from build123d import *

# Parameters (mm, degrees)
SKETCH_1_R          = 10
EXTRUDE_1_DEPTH     = 2
SKETCH_3_R          = 7.5
CUT_EXTRUDE_1_DEPTH = 12.5
SKETCH_5_R          = 1
SKETCH_5_W          = 2
SKETCH_5_H          = 2
EXTRUDE_5_DEPTH     = 1.5


with BuildPart() as part:
    # 草图1 → 凸台-拉伸1 (new body)
    with BuildSketch(Plane(origin=(0, 0, 0), x_dir=(0, 0, -1), z_dir=(1, 0, 0))):
        Circle(SKETCH_1_R)
    extrude(amount=EXTRUDE_1_DEPTH)

    # 草图3 → 切除-拉伸1 (cut)
    with BuildSketch(Plane(origin=(2, 0, 0), x_dir=(0, 0, -1), z_dir=(1, 0, 0))):
        Circle(SKETCH_3_R)
    extrude(amount=-CUT_EXTRUDE_1_DEPTH, mode=Mode.SUBTRACT)

    # 草图5 → 凸台-拉伸5 (add)
    with BuildSketch(Plane(origin=(2, 0, 0), x_dir=(0, 0, -1), z_dir=(1, 0, 0))):
        with Locations((0, 8.5)):
            Circle(SKETCH_5_R)
        with Locations((7.361215932, -4.25)):
            Circle(SKETCH_5_R)
        with Locations((-7.361215932, -4.25)):
            Circle(SKETCH_5_R)
        with Locations((-5.629165125, -3.25)):
            Circle(SKETCH_5_R)
        with Locations((0, 6.5)):
            Circle(SKETCH_5_R)
        with Locations((5.629165125, -3.25)):
            Circle(SKETCH_5_R)
        Polygon((-7.861215932, -3.383974596), (-6.129165125, -2.383974596), (-5.129165125, -4.116025404), (-6.861215932, -5.116025404), align=None)
        with Locations((0, 7.5)):
            Rectangle(SKETCH_5_W, SKETCH_5_H)
        Polygon((6.129165125, -2.383974596), (7.861215932, -3.383974596), (6.861215932, -5.116025404), (5.129165125, -4.116025404), align=None)
    extrude(amount=EXTRUDE_5_DEPTH)


solid = part.part
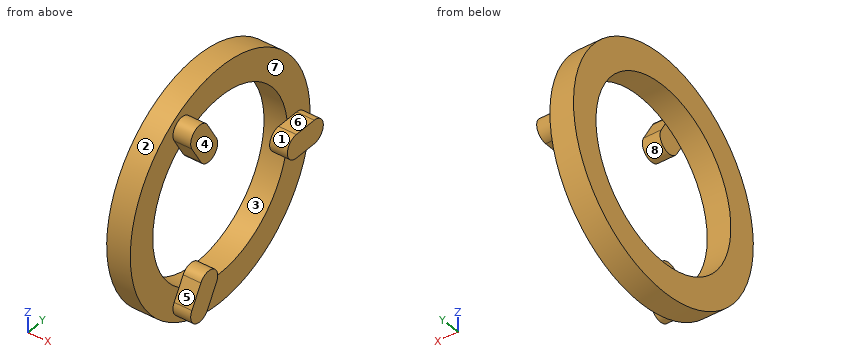
Part model, mm, in its own coordinate system. Face numbers are marked on the shaded views. A direction names the side the tool comes from. Coordinates: 2 decimals unless noted, no trailing zeros. Loops run counter-clockwise (first coordinate to the right, second up) from the corner with the lowest first, then second, coordinate; pieces in that order, holes last. Notation, with made-up numbers: (69.25, 55) -> (114.25, 55) arc R27 cw to (114.25, 76) -> close; hole circle Ø4 at (84.25, 61). An arc over 180 degrees is marked (long way). Use a Markdown table: item, result. Add a question column.
Item 1: Band-saw the part on D-D on x = 1.4. Write the cut outline in (y, z), plus the area to 3 significant figures.
Item 2: Band-saw the part on B-B on x = 3.1. Write the cut outline in (y, z), plus the area to 3 significant figures.
Item 3: Pull direction Y, two halves, no side cores. Call the marked faces 1, 2 and 3: +Y half, -Y half, draft (parallel to the pull), parting line (faces both ways), or undercut.
Item 4: Band-saw the part on C-C on z = 0. Write the cut outline in (x, y), plus the area to 3 significant figures.
Item 5: Probe probe 1 along Y at (x, z) = (1.05, 0); probe 2 along Z at (x, y) = (0.8, 2.5). List the from-to ranges inside material, lowest first.
Item 6: Which spindle directions (+Z, -Z, +X, -X, +Y, -Y) get a long thin tool onto all of the face, cutting with end or side? Do the marked faces 4, 5, 6, 7 and 8. Say none if no direction does.
Item 7: Band-saw the part on A-A on y = 0. Write the cut outline in (x, z), plus the area to 3 significant figures.
Item 8: Flat gauge pins, fed straight in: P1, Ø1.2, axis at x = 3, y = 7, coming from the +Z side; P2, Ø1.2, axis at y = -3, z = -6, coming from the -X side; P3, Ø1, axis at x = 1.5, z = 2.5, coming from the -Y side. Where does each tip first touch, or does it go through?
Geometry says:
| question | item | result |
|---|---|---|
| 1 | outline | circle Ø20 at (0, 0); hole circle Ø15 at (0, 0) |
| 1 | area | 137 mm² |
| 2 | outline | (-5.12, -6.86) arc R1 ccw to (-3.38, -7.86) -> (-2.38, -6.13) arc R1 ccw to (-4.12, -5.13) -> close; (-5.12, 6.86) -> (-4.12, 5.13) arc R1 ccw to (-2.38, 6.13) -> (-3.38, 7.86) arc R1 ccw to start; (6.5, -1) -> (8.5, -1) arc R1 ccw to (8.5, 1) -> (6.5, 1) arc R1 ccw to start |
| 2 | area | 21.4 mm² |
| 3 | face 1 | -Y half |
| 3 | face 2 | parting line |
| 3 | face 3 | undercut |
| 4 | outline | (0, -10) -> (2, -10) -> (2, -7.5) -> (0, -7.5) -> close; (0, 7.5) -> (2, 7.5) -> (2, 5.5) -> (3.5, 5.5) -> (3.5, 9.5) -> (2, 9.5) -> (2, 10) -> (0, 10) -> close |
| 4 | area | 16.0 mm² |
| 5 | probe 1 | -10 to -7.5, 7.5 to 10 |
| 5 | probe 2 | -9.68 to -7.07, 7.07 to 9.68 |
| 6 | face 4 | +Z, -Z, +X, +Y, -Y |
| 6 | face 5 | +X, -Y |
| 6 | face 6 | +Z, +X, +Y, -Y |
| 6 | face 7 | +X |
| 6 | face 8 | +X, -X |
| 7 | outline | (0, -10) -> (2, -10) -> (2, -7.5) -> (0, -7.5) -> close; (0, 7.5) -> (2, 7.5) -> (2, 10) -> (0, 10) -> close |
| 7 | area | 10.0 mm² |
| 8 | P1 | z = 1 |
| 8 | P2 | x = 2 |
| 8 | P3 | y = -9.8 |
